The drawing under review shows one solid part. Ordinate dimensions are in mm from its lowest x, y, z. A direction names the side the tool comes from. Give positions to 0.01 mm unless a question says otherwise; leave off trailing zeros. Write each loop counter-clockwise with the first axis right and the second up, starting at its lowest first coordinate (ties: lowest second). Pieces come first, ordered by that corner, then holes. Notation, with made-up numbers: (26, 54) -> (80, 54) arc R28 ccw to (80, 74) -> close; hole circle Ø2 at (66, -1). An arc over 180 degrees is marked (long way). Use CSV: the item, a comma, the result in double quotes.
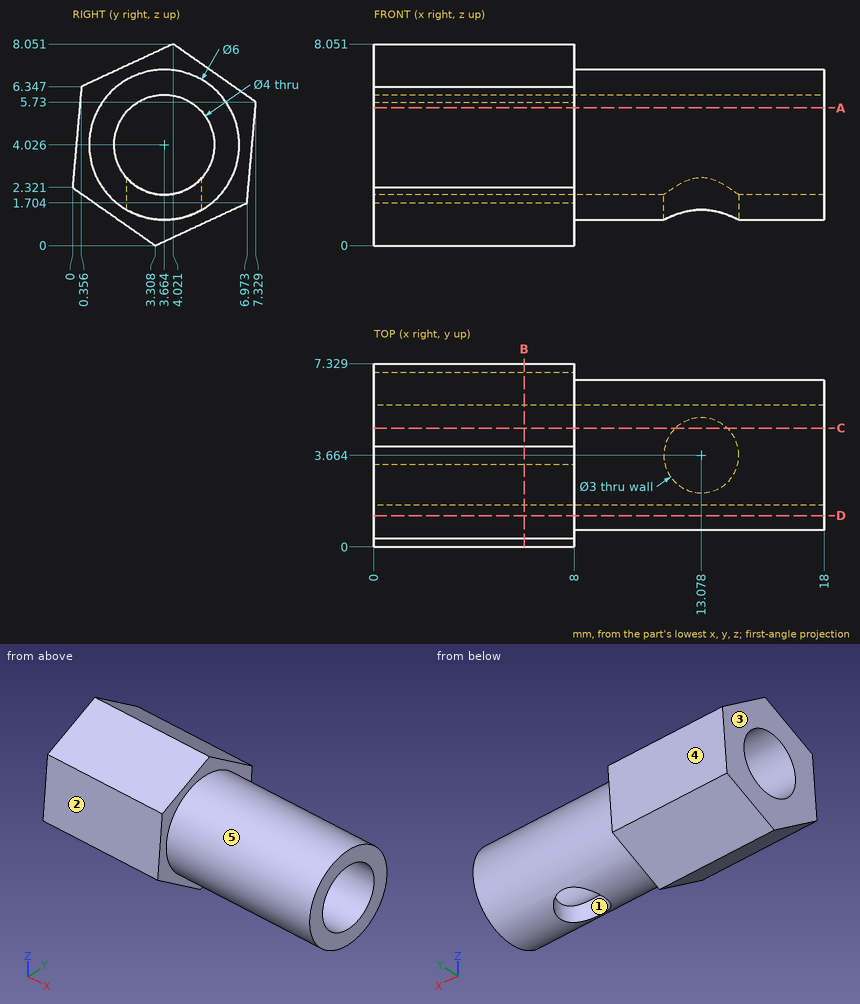
(1) Mouldability with a two-part tool opening along X and no side actions: class the marked faces 1, 2 and 3 as +X half, -X half, draft (parallel to the pull), parting line (faces both ways), or undercut.
Established:
face 1,"undercut"
face 2,"draft"
face 3,"-X half"
(2) Take a section at B-B (x = 6). Write out the cut boundary in (y, z) (1 decimal).
Established:
outline,"(0, 2.3) -> (3.3, 0) -> (7, 1.7) -> (7.3, 5.7) -> (4, 8.1) -> (0.4, 6.3) -> close; hole circle Ø4 at (3.7, 4)"
(3) Take a section at D-D (y = 1.25). Write out the cut boundary in (x, z) (1 decimal).
Established:
outline,"(0, 1.4) -> (8, 1.4) -> (8, 2.2) -> (18, 2.2) -> (18, 5.8) -> (8, 5.8) -> (8, 6.8) -> (0, 6.8) -> close"
(4) Tool access review of the marked faces 4 and 5: name each direction out of +Z, -Z, +X, -X, +Y, -Y from which nothing blocks a thin tool from reaching the whole face with its end or side.
Established:
face 4,"-Z, +X, -X, +Y"
face 5,"+X"
(5) Clearance check with flat-ended pins moving along their axes: pin 1 (1.8 mm diameter, centred on x = 13.08, y = 3.66, fed in from -Z); pin 2 (2 mm diameter, centred on y = 3.5, z = 2.5, fed in from +X). State where each tip first meets the part, or that it passes through.
Established:
pin 1,"stops at z = 5.81"
pin 2,"stops at x = 18"
(6) Take a section at A-A (z = 5.5). Write out the cut boundary in (x, y).
Established:
outline,"(0, 0.28) -> (8, 0.28) -> (8, 1.05) -> (18, 1.05) -> (18, 2.31) -> (0, 2.31) -> close; (0, 5.02) -> (18, 5.02) -> (18, 6.28) -> (8, 6.28) -> (8, 7.31) -> (0, 7.31) -> close"
(7) For line 1 along Y through (x, z) = (15.25, 4) (1 decimal); line 2 along X through (y, z) = (6.5, 2); line 3 along Y through (x, z) = (16, 3.75) (1 decimal), list the stretches that pass through material, from the lowest coordinate up. Write a range as [from, to].
Established:
line 1,"y = [0.7, 1.7], [5.7, 6.7]"
line 2,"x = [0, 8]"
line 3,"y = [0.7, 1.7], [5.6, 6.7]"
(8) Take a section at C-C (y = 4.75). Write out the cut boundary in (x, z) (1 decimal).
Established:
outline,"(0, 0.7) -> (8, 0.7) -> (8, 1.2) -> (12, 1.2) -> (12, 2.3) -> (0, 2.3) -> close; (0, 5.7) -> (18, 5.7) -> (18, 6.8) -> (8, 6.8) -> (8, 7.5) -> (0, 7.5) -> close; (14.1, 1.2) -> (18, 1.2) -> (18, 2.3) -> (14.1, 2.3) -> close"
